Work out the finished part from the listing and answer in its coordinate system (mm). Face numbers are marked on the shaded views. A direction names the side the tool comes from. Coordinates: 2 decimals unless noted, no trailing zeros. Loops run counter-clockwise (first coordinate to the right, second up) from the corner with the lowest first, then second, coordinate; pieces in that order, holes last. Notation, with made-up numbers: (29, 74.25) -> (52, 74.25) arc R26 ccw to (52, 102.25) -> close; hole circle Ø9 at (41, -34). An arc over 180 degrees is marked (long way). Use a Markdown table: item, result.
from build123d import *

# Parameters (mm, degrees)
EXTRUDE_1_DEPTH     = 9
CUT_EXTRUDE_1_REACH = 44.367
SKETCH_3_W          = 19.10949688
SKETCH_3_H          = 7.850581447
SKETCH_3_W_2        = 21.646823843
SKETCH_3_H_2        = 9.928676536
CUT_EXTRUDE_2_DEPTH = 43.367440329
SKETCH_5_W          = 6
SKETCH_5_H          = 9.57
CUT_EXTRUDE_3_DEPTH = 10
FILLET_1_R          = 2


with BuildPart() as part:
    # 草图1 → 凸台-拉伸1 (new, symmetric)
    with BuildSketch(Plane.XY):
        Polygon((-14, 33), (-2, 33), (0, 31), (0, 27.5), (-4, 27.5), (-4, 23), (0, 23), (0, 0), (-25, 0), (-25, 23), (-12, 23), (-12, 27.5), (-16, 27.5), (-16, 31), align=None)
    extrude(amount=EXTRUDE_1_DEPTH, both=True)

    # 切除-拉伸1: up to this face of the body (flat: up to its plane)
    cut_extrude_1_end = Plane(part.part.faces().sort_by_distance((-18.5, 23, 0))[0])
    # 草图3 → 切除-拉伸1 (cut, up to the picked face)
    with BuildSketch(Plane(origin=(0, 33, 0), x_dir=(1, 0, 0), z_dir=(0, 1, 0)), mode=Mode.PRIVATE) as cut_extrude_1_sk1:
        with Locations((-9.55474844, 8.075290724)):
            Rectangle(SKETCH_3_W, SKETCH_3_H)
    cut_extrude_1_tool1 = split(extrude(cut_extrude_1_sk1.sketch, amount=-CUT_EXTRUDE_1_REACH, mode=Mode.PRIVATE), bisect_by=cut_extrude_1_end, keep=Keep.BOTH, mode=Mode.PRIVATE)
    # 草图3 → 切除-拉伸1 (cut, up to the picked face)
    with BuildSketch(Plane(origin=(0, 33, 0), x_dir=(1, 0, 0), z_dir=(0, 1, 0)), mode=Mode.PRIVATE) as cut_extrude_1_sk2:
        with Locations((-8.286084959, -9.114338268)):
            Rectangle(SKETCH_3_W_2, SKETCH_3_H_2)
    cut_extrude_1_tool2 = split(extrude(cut_extrude_1_sk2.sketch, amount=-CUT_EXTRUDE_1_REACH, mode=Mode.PRIVATE), bisect_by=cut_extrude_1_end, keep=Keep.BOTH, mode=Mode.PRIVATE)
    add(cut_extrude_1_tool1.solids().sort_by(Axis((-9.554748, 33, -8.075291), (0, -1, 0)))[0], mode=Mode.SUBTRACT)
    add(cut_extrude_1_tool2.solids().sort_by(Axis((-8.286085, 33, 9.114338), (0, -1, 0)))[0], mode=Mode.SUBTRACT)

    # 草图4 → 切除-拉伸2 (cut, through all)
    with BuildSketch(Plane(origin=(0, 0, 0), x_dir=(0, 0, -1), z_dir=(1, 0, 0))):
        with BuildLine():
            Line((-3.25, 8.5), (-3.25, 14.5))
            ThreePointArc((-3.25, 14.5), (0, 17.75), (3.25, 14.5))
            Line((3.25, 14.5), (3.25, 8.5))
            ThreePointArc((3.25, 8.5), (0, 5.25), (-3.25, 8.5))
        make_face()
    extrude(amount=-CUT_EXTRUDE_2_DEPTH, mode=Mode.SUBTRACT)

    # 草图5 → 切除-拉伸3 (cut)
    with BuildSketch(Plane.XY.offset(9)):
        with Locations((-9.5, 11.5)):
            Rectangle(SKETCH_5_W, SKETCH_5_H)
    extrude(amount=-CUT_EXTRUDE_3_DEPTH, mode=Mode.SUBTRACT)

    # 圆角1
    fillet_1_edges = [part.edges().sort_by_distance(p)[0] for p in [
        (-12.5, 23, -9),
        (-12.5, 0, -9),
        (-12.5, 23, 9),
        (-12.5, 0, 9),
    ]]
    fillet(fillet_1_edges, radius=FILLET_1_R)


solid = part.part
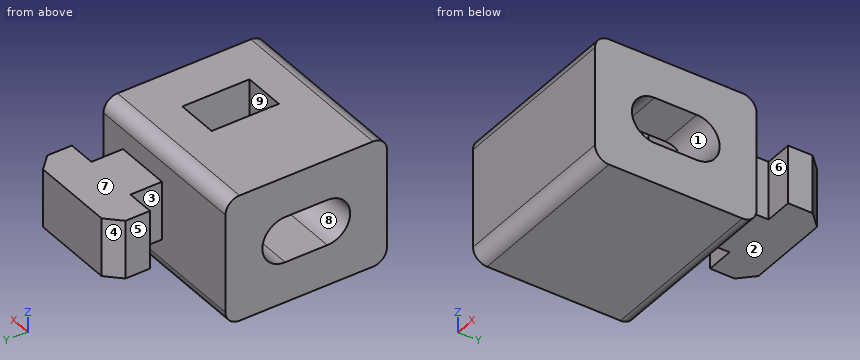
Q1. Consider line 1 (Z direction, x = -1.75, y = 9); line 2 (Y direction, x = -8.5, z = 7) (3 decimals); line 3 (Y direction, x = -9, z = -6.25). Determine where each line is inside the solid, lowest interval first. Write a range as [from, to].
Solved:
| item | result |
|---|---|
| line 1 | [-9, -3.25], [3.25, 9] |
| line 2 | [0, 6.715], [16.285, 23] |
| line 3 | [0, 23] |
Q2. Section B-B on z = -1.25 is taken. Determine the outline of the cut face in (x, y).
Solved:
| item | result |
|---|---|
| outline | (-25, 0) -> (0, 0) -> (0, 5.5) -> (-25, 5.5) -> close; (-25, 17.5) -> (0, 17.5) -> (0, 23) -> (-4, 23) -> (-4, 27.5) -> (0, 27.5) -> (0, 31) -> (-2, 33) -> (-14, 33) -> (-16, 31) -> (-16, 27.5) -> (-12, 27.5) -> (-12, 23) -> (-25, 23) -> close |
Q3. Section D-D on x = -18.5 is taken. Determine the outline of the cut face in (y, z), and give its area (3 significant figures).
Solved:
| item | result |
|---|---|
| outline | (0, -7) arc R2 ccw to (2, -9) -> (21, -9) arc R2 ccw to (23, -7) -> (23, 7) arc R2 ccw to (21, 9) -> (2, 9) arc R2 ccw to (0, 7) -> close; hole (8.5, -3.25) -> (14.5, -3.25) arc R3.25 ccw to (14.5, 3.25) -> (8.5, 3.25) arc R3.25 ccw to start |
| area | 338 mm² |
Q4. Section A-A on x = -15 is taken. Determine the outline of the cut face in (y, z).
Solved:
| item | result |
|---|---|
| outline | (0, -7) arc R2 ccw to (2, -9) -> (21, -9) arc R2 ccw to (23, -7) -> (23, 7) arc R2 ccw to (21, 9) -> (2, 9) arc R2 ccw to (0, 7) -> close; (27.5, -4.15) -> (32, -4.15) -> (32, 4.15) -> (27.5, 4.15) -> close; hole (8.5, -3.25) -> (14.5, -3.25) arc R3.25 ccw to (14.5, 3.25) -> (8.5, 3.25) arc R3.25 ccw to start |
Q5. Section C-C on z = 5 is taken. Determine the outline of the cut face in (x, y) (3 decimals), and give its area (3 significant figures).
Solved:
| item | result |
|---|---|
| outline | (-25, 0) -> (0, 0) -> (0, 23) -> (-25, 23) -> close; hole (-12.5, 6.715) -> (-6.5, 6.715) -> (-6.5, 16.285) -> (-12.5, 16.285) -> close |
| area | 518 mm² |
Q6. For the marked faces 5, 6, 7, 8 and 9, determine the directions among +Z, -Z, +X, -X, +Y, -Y from which every point of the face is accessible in a straight line to the end or side of a thin tool.
Solved:
| item | result |
|---|---|
| face 5 | +Z, -Z, -X, +Y |
| face 6 | +Z, -Z, +X |
| face 7 | +Z, +X, -X, +Y |
| face 8 | +X, -X |
| face 9 | +Z |
Q7. Determine the mould class of the marked faces 1, 2, 3 and 4 for opening direction Y: pulls with the +Y half, pulls with the -Y half, needs draft (parallel to the pull), parting line crosses it, or undercut.
Solved:
| item | result |
|---|---|
| face 1 | undercut |
| face 2 | needs draft |
| face 3 | undercut |
| face 4 | pulls with the +Y half |
Q8. Given pin 1 Ø2 at (y, z) = (24.5, 1.5) entering from +X; pin 2 Ø1.8 at (y, z) = (28.5, -0.5) entering from -X; pin 3 Ø1 at (x, z) = (-9, 6) entering from +Y, each flat-ended and moving along its own axis, determine where each tip first touches the part or whether it passes through.
Solved:
| item | result |
|---|---|
| pin 1 | x = -4 |
| pin 2 | x = -16 |
| pin 3 | y = 23 |
